```python
from build123d import *

# Parameters (mm, degrees)
F0_W      = 609.6
F0_H      = 457.2
F1_DEPTH  = 50.8
F2_W      = 76.2
F2_H      = 76.2
F3_DEPTH  = 711.2
F4_W      = 203.2
F4_H      = 101.6
F5_DEPTH  = 25.4
F6_R      = 5.980424
F7_DEPTH  = 25.4
F8_W      = 38.1
F8_H      = 38.1
F9_DEPTH  = 457.2
F10_W     = 38.1
F10_H     = 38.1
F11_DEPTH = 152.4
F12_W     = 6.35
F12_H     = 38.1
F13_DEPTH = 76.2
F14_R     = 9
F15_DEPTH = 25.4


with BuildPart() as f1:
    # F0 (on Top) → F1 (new body)
    with BuildSketch(Plane.XY):
        Rectangle(F0_W, F0_H)
    extrude(amount=F1_DEPTH)

    # F2 (on face) → F3 (join)
    with BuildSketch(Plane.XY.offset(50.8)):
        with Locations((38.1, 8.698421)):
            Rectangle(F2_W, F2_H)
    extrude(amount=F3_DEPTH)

    # F4 (on face) → F5 (join)
    with BuildSketch(Plane.XY.offset(762)):
        with Locations((12.7, 8.698421)):
            Rectangle(F4_W, F4_H)
    extrude(amount=F5_DEPTH)

    # F6 (on face) → F7 (cut)
    with BuildSketch(Plane.XY.offset(787.4)):
        with Locations((-76.2, 46.798421)):
            Circle(F6_R)
        with Locations((-76.2, 21.398421)):
            Circle(F6_R)
        with Locations((-76.2, -4.001579)):
            Circle(F6_R)
        with Locations((-76.2, -29.401579)):
            Circle(F6_R)
        with Locations((-50.8, 46.798421)):
            Circle(F6_R)
        with Locations((-50.8, 21.398421)):
            Circle(F6_R)
        with Locations((-50.8, -4.001579)):
            Circle(F6_R)
        with Locations((-50.8, -29.401579)):
            Circle(F6_R)
        with Locations((-25.4, 46.798421)):
            Circle(F6_R)
        with Locations((-25.4, 21.398421)):
            Circle(F6_R)
        with Locations((-25.4, -4.001579)):
            Circle(F6_R)
        with Locations((-25.4, -29.401579)):
            Circle(F6_R)
        with Locations((0, 46.798421)):
            Circle(F6_R)
        with Locations((0, 21.398421)):
            Circle(F6_R)
        with Locations((0, -4.001579)):
            Circle(F6_R)
        with Locations((0, -29.401579)):
            Circle(F6_R)
        with Locations((25.4, 46.798421)):
            Circle(F6_R)
        with Locations((25.4, 21.398421)):
            Circle(F6_R)
        with Locations((25.4, -4.001579)):
            Circle(F6_R)
        with Locations((25.4, -29.401579)):
            Circle(F6_R)
        with Locations((50.8, 46.798421)):
            Circle(F6_R)
        with Locations((50.8, 21.398421)):
            Circle(F6_R)
        with Locations((50.8, -4.001579)):
            Circle(F6_R)
        with Locations((50.8, -29.401579)):
            Circle(F6_R)
        with Locations((76.2, 46.798421)):
            Circle(F6_R)
        with Locations((76.2, 21.398421)):
            Circle(F6_R)
        with Locations((76.2, -4.001579)):
            Circle(F6_R)
        with Locations((76.2, -29.401579)):
            Circle(F6_R)
        with Locations((101.6, 46.798421)):
            Circle(F6_R)
        with Locations((101.6, 21.398421)):
            Circle(F6_R)
        with Locations((101.6, -4.001579)):
            Circle(F6_R)
        with Locations((101.6, -29.401579)):
            Circle(F6_R)
    extrude(amount=-F7_DEPTH, mode=Mode.SUBTRACT)

    # F8 (on face) → F9 (join)
    with BuildSketch(Plane.YZ.offset(76.2)):
        with Locations((19.05, 527.05)):
            Rectangle(F8_W, F8_H)
    extrude(amount=F9_DEPTH)

    # F10 (on face) → F11 (join)
    with BuildSketch(Plane.XY.offset(546.1)):
        with Locations((514.35, 19.05)):
            Rectangle(F10_W, F10_H)
    extrude(amount=F11_DEPTH)

    # F12 (on face) → F13 (join)
    with BuildSketch(Plane.XY.offset(698.5)):
        with Locations((530.225, 19.05)):
            Rectangle(F12_W, F12_H)
    extrude(amount=F13_DEPTH)

    # F14 (on face) → F15 (cut)
    with BuildSketch(Plane.YZ.offset(533.4)):
        with Locations((19.05, 749.3)):
            Circle(F14_R)
    extrude(amount=-F15_DEPTH, mode=Mode.SUBTRACT)


solid = f1.part
```
Model file for the job. Use its own axes, mm. A direction names the side the tool comes from. Coordinates: 2 decimals unless noted, no trailing zeros. Write each loop counter-clockwise with the first axis right and the second up, starting at its lowest first coordinate (ties: lowest second). Pieces come first, ordered by that corner, then holes. Notation, with made-up numbers: (-0.5, 76) - (56.5, 76) arc R29 ccw to (56.5, 113) - close; hole circle Ø6 at (68.5, -4.5). An arc over 180 degrees is marked (long way). One line per item, written item: value. Start each with the question number.
1. Mould opens along Z. For faces 4 (the flat face through (0, 8, 401)), 5 (the flat face through (511, 19, 698.5)), 6 (the flat face through (527.05, 19, 736)) say: released by +Z, released by -Z, zero draft, split by the parting line, or undercut.
2. Slice it at A-A (x = 233.5). Write the cut outline in (y, z).
3. Slice it at D-D (z = 173.5). Write the cut outline in (x, y).
4. Slice it at C-C (y = -125). Write the cut outline in (x, z).
5. Probe line 1 (Y direction, x = 0, z = 778.75); line 2 (Z direction, x = 114, y = 22); line 3 (Y direction, x = 101, z = 773). List the from-to ranges inside material, lowest first. Write a range as from..to.
6. Tool access for faces 1 (the flat face through (38, -29.402, 401)), 2 (the flat face through (38, 46.798, 401)), 3 (the flat face through (-88.9, 8, 775)): list every direction of +Z, -Z, +X, -X, +Y, -Y with a clear straight run to the whole face (end or side of a thin tool).
7. Slice it at B-B (z = 616). Write the cut outline in (x, y), plus the area to 3 significant figures.
8. Flat gauge pins, fed straight in: pin 1 (11 mm diameter, centred on x = -25.4, y = 21.4, fed in from +Z); pin 2 (1.9 mm diameter, centred on x = 530, y = 16.5, fed in from +Z); pin 3 (6.5 mm diameter, centred on x = 74, y = 22, fed in from +Z). Where does each tip first touch, or does it go through?
Answers below:
1. face 4: undercut
1. face 5: released by +Z
1. face 6: zero draft
2. outline: (-228.6, 0) - (228.6, 0) - (228.6, 50.8) - (-228.6, 50.8) - close; (0, 508) - (38.1, 508) - (38.1, 546.1) - (0, 546.1) - close
3. outline: (0, -29.4) - (76.2, -29.4) - (76.2, 46.8) - (0, 46.8) - close
4. outline: (-304.8, 0) - (304.8, 0) - (304.8, 50.8) - (-304.8, 50.8) - close
5. line 1: y = -42.1..-35.38, -23.42..-9.98, 1.98..15.42, 27.38..40.82, 52.78..59.5
5. line 2: z = 0..50.8, 508..546.1, 762..787.4
5. line 3: y = -42.1..-35.35, -23.45..-9.95, 1.95..15.45, 27.35..40.85, 52.75..59.5
6. face 1: +X, -X, -Y
6. face 2: +X, -X, +Y
6. face 3: +Z, -X, +Y, -Y
7. outline: (0, -29.4) - (76.2, -29.4) - (76.2, 46.8) - (0, 46.8) - close; (495.3, 0) - (533.4, 0) - (533.4, 38.1) - (495.3, 38.1) - close
7. area: 7,260 mm^2
8. pin 1: stops at z = 50.8
8. pin 2: stops at z = 774.7
8. pin 3: stops at z = 762
